The model under review builds one solid part; all positions refer to its coordinate system, in mm. A direction names the side the tool comes from. Round coordinates to 2 decimals unless told otherwise and drop trailing zeros. Loops run counter-clockwise (first coordinate to the right, second up) from the corner with the lowest first, then second, coordinate; pieces in that order, holes last. Notation, with made-up numbers: (28, 43.25) - (43, 43.25) arc R22 ccw to (43, 61.25) - close; hole circle Ø7 at (51, -5.5). An arc over 180 degrees is marked (long way). Answer as CSV lines item,"result".
from build123d import *

# Parameters (mm, degrees)
SKETCH1_R           = 9
SKETCH1_R_2         = 3.525
BOSS_EXTRUDE1_DEPTH = 6
SKETCH2_W           = 7.05
SKETCH2_H           = 1.05
BOSS_EXTRUDE2_DEPTH = 6
SKETCH3_R           = 1.55
CUT_EXTRUDE1_DEPTH  = 8
CIRPATTERN1_COUNT   = 4


with BuildPart() as part:
    # Sketch1 → Boss-Extrude1 (new body)
    with BuildSketch(Plane(origin=(0, 0, 0), x_dir=(1, 0, 0), z_dir=(0, 1, 0))):
        Circle(SKETCH1_R)
        Circle(SKETCH1_R_2, mode=Mode.SUBTRACT)
    extrude(amount=BOSS_EXTRUDE1_DEPTH)

    # Sketch2 → Boss-Extrude2 (add)
    with BuildSketch(Plane(origin=(0, 0, 0), x_dir=(1, 0, 0), z_dir=(0, 1, 0))):
        Rectangle(SKETCH2_W, SKETCH2_H)
    extrude(amount=BOSS_EXTRUDE2_DEPTH)

    # Sketch3 → Cut-Extrude1 (cut)
    with BuildSketch(Plane(origin=(0, 6, 0), x_dir=(1, 0, 0), z_dir=(0, 1, 0))):
        with Locations((6, 0)):
            Circle(SKETCH3_R)
    cut_extrude1 = extrude(amount=-CUT_EXTRUDE1_DEPTH, mode=Mode.SUBTRACT)

    # CirPattern1: Cut-Extrude1 ×4 about axis
    cirpattern1_axis = Axis((0, 0, 0), (0, 1, 0))
    for i in range(1, CIRPATTERN1_COUNT):
        add(cut_extrude1.rotate(cirpattern1_axis, i * 360 / CIRPATTERN1_COUNT), mode=Mode.SUBTRACT)


solid = part.part
1. Draft analysis for pull direction X (two halves, no side actions). For faces 3 (the face through (-1.172, 2.958, -8.923)), 4 (the face through (0, 3, 0.525)), 5 (the face through (0, 6, 0)), state which applies: +X half, -X half, draft (parallel to the pull), parting line (faces both ways), or undercut.
Numbers:
face 3,"parting line"
face 4,"undercut"
face 5,"draft"
2. Take a section at A-A (x = 0). State the section outline as (y, z) points (3 decimals).
Numbers:
outline,"(0, -9) - (6, -9) - (6, -7.55) - (0, -7.55) - close; (0, -4.45) - (6, -4.45) - (6, -3.525) - (0, -3.525) - close; (0, -0.525) - (6, -0.525) - (6, 0.525) - (0, 0.525) - close; (0, 3.525) - (6, 3.525) - (6, 4.45) - (0, 4.45) - close; (0, 7.55) - (6, 7.55) - (6, 9) - (0, 9) - close"
3. Tool access review of faces 1 (the face through (0, 3, -0.525)), 2 (the face through (0, 0, 0)): name each direction out of +Z, -Z, +X, -X, +Y, -Y from which nothing blocks a thin tool from reaching the whole face with its end or side.
Numbers:
face 1,"+Y, -Y"
face 2,"+Z, -Z, +X, -X, -Y"
4. Clearance check with flat-ended pins moving along their axes: pin 1 (3 mm diameter, centred on x = -5, y = 5, fed in from -Z); pin 2 (2 mm diameter, centred on y = 4, z = -5.5, fed in from +X); pin 3 (1 mm diameter, centred on x = -6.5, y = 3.5, fed in from -Z). State where each tip first meets the part, or that it passes through.
Numbers:
pin 1,"stops at z = -8.29"
pin 2,"stops at x = 7.79"
pin 3,"stops at z = -6.71"
5. Take a section at D-D (x = 7). State the section outline as (y, z) points.
Numbers:
outline,"(0, -5.66) - (6, -5.66) - (6, -1.18) - (0, -1.18) - close; (0, 1.18) - (6, 1.18) - (6, 5.66) - (0, 5.66) - close"
6. Take a section at B-B (y = 5.05). State the section outline as (x, z) points (3 decimals).
Numbers:
outline,"circle Ø18 at (0, 0); hole circle Ø3.1 at (-6, 0); hole (-3.486, -0.525) arc R3.525 ccw to (3.486, -0.525) - close; hole (-3.486, 0.525) - (3.486, 0.525) arc R3.525 ccw to start; hole circle Ø3.1 at (0, -6); hole circle Ø3.1 at (0, 6); hole circle Ø3.1 at (6, 0)"
7. Take a section at C-C (z = 5.5). State the section outline as (x, y) points, plus the area to 3 significant figures.
Numbers:
outline,"(-7.12, 0) - (-1.47, 0) - (-1.47, 6) - (-7.12, 6) - close; (1.47, 0) - (7.12, 0) - (7.12, 6) - (1.47, 6) - close"
area,"67.9 mm²"
8. Wall thickness on probe 1 along Z at (x, y) = (-3.25, 3.1) (3 decimals); probe 2 along Z at (x, y) = (0.25, 2.85) (3 decimals); probe 3 along X at (y, z) = (2.75, -6.5): over which ranges is each line inside the solid? List them lowest first.
Numbers:
probe 1,"z = -8.393 to -1.365, -0.525 to 0.525, 1.365 to 8.393"
probe 2,"z = -8.997 to -7.53, -4.47 to -3.516, -0.525 to 0.525, 3.516 to 4.47, 7.53 to 8.997"
probe 3,"x = -6.22 to -1.47, 1.47 to 6.22"
